Check sheet for the modelled part. Datum: model origin and axes. Units: mm. Round coordinates to 2 decimals unless told otherwise and drop trailing zeros.
Autodesk Fusion 360 part; units mm, degrees
sketch "Sketch1" plane through (0, 0, 0) normal (0, 1, 0) x (1, 0, 0)
  line L0 (-71.0683, 54.7697) -> (72.9317, 54.7697)
  line L1 (72.9317, 54.7697) -> (72.9317, -52.2303)
  line L2 (-71.0683, -56.2303) -> (-71.0683, 54.7697)
  line L3 (-2.0683, -56.2303) -> (-2.0683, -55.2303)
  line L4 (-2.0683, -55.2303) -> (43.9317, -55.2303)
  line L5 (43.9317, -55.2303) -> (43.9317, -56.2303)
  line L6 (68.9317, -56.2303) -> (43.9317, -56.2303)
  line L7 (-2.0683, -56.2303) -> (-71.0683, -56.2303)
  line L8 (72.9317, -52.2303) -> (68.9317, -52.2303) construction
  line L9 (68.9317, -56.2303) -> (68.9317, -52.2303) construction
  line L10 (68.9317, -56.2303) -> (72.9317, -52.2303)
  circle A0 centre (-63.0683, -11.2303) radius 1.5
  circle A1 centre (26.9317, 41.7697) radius 1.5
  dimension "d3" = 1
  dimension "d4" = 46
  dimension "d5" = 69
  dimension "d6" = 4
  dimension "d8" = 4
  dimension "d11" = 4
  dimension "d14" = 144
  dimension "d17" = 25
  dimension "d18" = 3
  dimension "d19" = 8
  dimension "d20" = 66
  dimension "d21" = 111
  dimension "d23" = 111
  dimension "d24" = 45
  dimension "d25" = 3
  dimension "d26" = 13
  dimension "d27" = 46
  dimension "d28" = 98
extrude "Extrude1" add sketch "Sketch1" along normal blind 1.6
1) Draft check along X on faces 1 (the face through (28.362, 0.789, -41.319)), 2 (the face through (70.9, 0.79, 54.26)), 3 (the face through (0, 0, 0)). Enter one of: pulls with the +X half, pulls with the -X half, needs draft (parallel to the pull), parting line crosses it, or undercut.
2) Scan lines: line 1 (X direction, y = 1, z = 12); line 2 (Z direction, x = 7.5, y = 1.2). Record each from-to range of solid material in increasing order.
3) Gauge pin test, flat end, axial feed: pin 1 (0.8 mm diameter, centred on x = 27.5, y = 0.5, fed in from +Z). Record the tip position at first contact, or that the pin passes through.
Values found:
1. face 1: undercut
1. face 2: pulls with the +X half
1. face 3: needs draft
2. line 1: x = -71.07 to -64.36, -61.78 to 72.93
2. line 2: z = -54.77 to 55.23
3. pin 1: stops at z = 55.23
